```python
from build123d import *

# Parameters (mm, degrees)
SKETCH3_R           = 63.5
SKETCH3_R_2         = 57.15
SKETCH3_W           = 60.426788384
SKETCH3_H           = 37.666233726
BOSS_EXTRUDE1_DEPTH = 6.35
SKETCH2_W           = 46.99
SKETCH2_H           = 26.67
CUT_EXTRUDE1_DEPTH  = 3.81
FILLET1_R           = 6.35
SKETCH6_W           = 35.970839212
SKETCH6_H           = 12.396108552
CUT_EXTRUDE2_DEPTH  = 6.35
FILLET2_R           = 5.08
SKETCH3_4_R         = 57.15
SKETCH3_4_W         = 60.426788384
SKETCH3_4_H         = 37.666233726
CUT_EXTRUDE4_DEPTH  = 3.81
FILLET3_R           = 5.08


with BuildPart() as part:
    # Sketch3 → Boss-Extrude1 (new body)
    # profile 1 of 3: a face of its own
    with BuildSketch(Plane.XY):
        Circle(SKETCH3_R)
        Circle(SKETCH3_R_2, mode=Mode.SUBTRACT)
    # profile 2 of 3: a face of its own
    with BuildSketch(Plane.XY):
        Circle(SKETCH3_R_2)
    # profile 3 of 3: a face of its own
    with BuildSketch(Plane.XY):
        with Locations((-11.125000102, 0)):
            Rectangle(SKETCH3_W, SKETCH3_H)
    extrude(amount=BOSS_EXTRUDE1_DEPTH)

    # Sketch2 → Cut-Extrude1 (cut)
    with BuildSketch(Plane.XY):
        with Locations((-11.125000102, 0)):
            Rectangle(SKETCH2_W, SKETCH2_H)
    extrude(amount=CUT_EXTRUDE1_DEPTH, mode=Mode.SUBTRACT)

    # Fillet1
    fillet1_edges = [part.edges().sort_by_distance(p)[0] for p in [
        (12.369999898, -13.335, 1.905),
        (12.369999898, 13.335, 1.905),
        (-34.620000102, 13.335, 1.905),
        (-34.620000102, -13.335, 1.905),
    ]]
    fillet(fillet1_edges, radius=FILLET1_R)

    # Sketch6 → Cut-Extrude2 (cut)
    with BuildSketch(Plane.XY):
        with Locations((-11.125000102, 0)):
            Rectangle(SKETCH6_W, SKETCH6_H)
    extrude(amount=CUT_EXTRUDE2_DEPTH, mode=Mode.SUBTRACT)

    # Fillet2
    fillet2_edges = [part.edges().sort_by_distance(p)[0] for p in [
        (6.860419504, -6.198054276, 5.08),
        (6.860419504, 6.198054276, 5.08),
        (-29.110419708, 6.198054276, 5.08),
        (-29.110419708, -6.198054276, 5.08),
    ]]
    fillet(fillet2_edges, radius=FILLET2_R)

    # Sketch3_4 → Cut-Extrude4 (cut)
    with BuildSketch(Plane.XY):
        with Locations(Location((0, 0, 0), (0, 0, 180))):
            Circle(SKETCH3_4_R)
        with Locations((-11.125000102, 0)):
            Rectangle(SKETCH3_4_W, SKETCH3_4_H, mode=Mode.SUBTRACT)
    extrude(amount=CUT_EXTRUDE4_DEPTH, mode=Mode.SUBTRACT)

    # Fillet3
    fillet3_edges = [part.edges().sort_by_distance(p)[0] for p in [
        (-41.338394294, 18.833116863, 1.905),
        (19.08839409, 18.833116863, 1.905),
        (19.08839409, -18.833116863, 1.905),
        (-41.338394294, -18.833116863, 1.905),
    ]]
    fillet(fillet3_edges, radius=FILLET3_R)


solid = part.part
```
Source: CAD feature listing. Evaluate the final solid. Frame: model axes, mm. A direction names the side the tool comes from. Coordinates: 2 decimals unless noted, no trailing zeros. Loops run counter-clockwise (first coordinate to the right, second up) from the corner with the lowest first, then second, coordinate; pieces in that order, holes last. Notation, with made-up numbers: M -34,56 L 3,56 A21 cw 3,67 Z; hole C 68.25,4 d8. An arc over 180 degrees is marked long. Use a Markdown table: item, result. Add a question column.
Q1. Material intervals for L1, parallel to Y at x = 0, z = 1.65 (3 decimals); L2, parallel to Y at x = -1, z = 4; L3, parallel to X at y = -5, z = 3.25, sorted ascending.
Q2. Section query B-B, the plane x = 0. Return loops of the section in (y, z) (3 decimals).
Q3. Draft query along Y for faces 4 (the cylindrical face through (-13.77, -61.99, 3.13)), 5 (the cylindrical face through (10.559, 11.425, 1.932)), 6 (the flat face through (-12, 17, 0)). Return one class per face: pulls with the +Y half, pulls with the -Y half, needs draft (parallel to the pull), parting line crosses it, or undercut.
Q4. Section query C-C, the plane y = 49. Return loops of the section in (x, z), and give its area (3 significant figures).
Q5. First-contact query: pin 1 (1.9 mm diameter, centred on y = -6.5, z = 1.5, fed in from +X); pin 2 (1.1 mm diameter, centred on x = -9, z = 2, fed in from +Y); pin 3 (2 mm diameter, centred on y = 37.5, z = 4, fed in from -X). Flat tips, straight axial feed; report the tip coordinate or a pass-through.
Q6. Access query for faces 1 (the flat face through (-57, 10, 0)), 2 (the flat face through (-41.338, 0, 2)), 3 (the cylindrical face through (-27.66, -4.67, 5.1)). Directions: +Z, -Z, +X, -X, +Y, -Y. A direction counts if a zero-diameter tool reaches every point of the face in a straight line with its end or side. Return the directions, or none.
Q7. Section query D-D, the plane x = 27. Return loops of the section in (y, z), and give its area (3 significant figures).
Q8. Section query A-A, the plane z = 1. Return loops of the section in (x, y) (3 decimals).
Result:
| question | item | result |
|---|---|---|
| 1 | L1 | y = -63.5 to -57.15, -18.833 to -13.335, 13.335 to 18.833, 57.15 to 63.5 |
| 1 | L2 | y = -63.49 to -6.2, 6.2 to 63.49 |
| 1 | L3 | x = -63.3 to -56.93, -41.34 to -34.62, 12.37 to 19.09, 56.93 to 63.3 |
| 2 | outline | M -63.5,0 L -57.15,0 L -57.15,3.81 L -18.833,3.81 L -18.833,0 L -13.335,0 L -13.335,3.81 L -6.198,3.81 L -6.198,6.35 L -63.5,6.35 Z; M 6.198,3.81 L 13.335,3.81 L 13.335,0 L 18.833,0 L 18.833,3.81 L 57.15,3.81 L 57.15,0 L 63.5,0 L 63.5,6.35 L 6.198,6.35 Z |
| 3 | face 4 | parting line crosses it |
| 3 | face 5 | undercut |
| 3 | face 6 | needs draft |
| 4 | outline | M -40.39,0 L -29.41,0 L -29.41,3.81 L 29.41,3.81 L 29.41,0 L 40.39,0 L 40.39,6.35 L -40.39,6.35 Z |
| 4 | area | 289 mm2 |
| 5 | pin 1 | stops at x = 63.26 |
| 5 | pin 2 | stops at y = 62.94 |
| 5 | pin 3 | stops at x = -51.96 |
| 6 | face 1 | -Z, +X, -X, +Y, -Y |
| 6 | face 2 | -Z |
| 6 | face 3 | +Z, -Z |
| 7 | outline | M -57.47,0 L -50.37,0 L -50.37,3.81 L 50.37,3.81 L 50.37,0 L 57.47,0 L 57.47,6.35 L -57.47,6.35 Z |
| 7 | area | 346 mm2 |
| 8 | outline | C 0,0 d127; M -41.338,-13.753 A5.08 ccw -36.258,-18.833 L 14.008,-18.833 A5.08 ccw 19.088,-13.753 L 19.088,13.753 A5.08 ccw 14.008,18.833 L -36.258,18.833 A5.08 ccw -41.338,13.753 Z; hole C 0,0 d114.3; hole M -34.62,-6.985 A6.35 ccw -28.27,-13.335 L 6.02,-13.335 A6.35 ccw 12.37,-6.985 L 12.37,6.985 A6.35 ccw 6.02,13.335 L -28.27,13.335 A6.35 ccw -34.62,6.985 Z |
